from build123d import *

# Parameters (mm, degrees)
SKETCH1_R           = 2.5
BOSS_EXTRUDE1_DEPTH = 1
SKETCH2_R           = 1.5
BOSS_EXTRUDE2_DEPTH = 11.75
BOSS_EXTRUDE3_START = -12.75
SKETCH1_5_R         = 2.5
BOSS_EXTRUDE3_DEPTH = 1
FILLET1_R           = 0.05
SCALE1_SCALE        = 1.9


with BuildPart() as part:
    # Sketch1 → Boss-Extrude1 (new body)
    with BuildSketch(Plane.XY):
        Circle(SKETCH1_R)
    extrude(amount=-BOSS_EXTRUDE1_DEPTH)

    # Sketch2 → Boss-Extrude2 (add)
    with BuildSketch(Plane(origin=(0, 0, -1), x_dir=(-1, 0, 0), z_dir=(0, 0, -1))):
        Circle(SKETCH2_R)
    extrude(amount=BOSS_EXTRUDE2_DEPTH)

    # Sketch1<5> → Boss-Extrude3 (add)
    with BuildSketch(Plane.XY.offset(BOSS_EXTRUDE3_START)):
        Circle(SKETCH1_5_R)
    extrude(amount=-BOSS_EXTRUDE3_DEPTH)

    # Fillet1
    fillet1_edges = [part.edges().sort_by_distance(p)[0] for p in [
        (-2.5, 0, 0),
        (-2.5, 0, -1),
        (-2.5, 0, -12.75),
        (-2.5, 0, -13.75),
    ]]
    fillet(fillet1_edges, radius=FILLET1_R)


with BuildPart() as part_1:
    # Scale1: scaled about (0, 0, -6.875)
    add(part.part.scale(SCALE1_SCALE).moved(Location((0, 0, 6.1875))))


solid = part_1.part
Can you work these out from the model? Positions are in its coordinate system, mm. A direction names the side the tool comes from. Round coordinates to 2 decimals unless told otherwise and drop trailing zeros. Loops run counter-clockwise (first coordinate to the right, second up) from the corner with the lowest first, then second, coordinate; pieces in that order, holes last. Notation, with made-up numbers: (67, 54) - (107, 54) arc R24 cw to (107, 71) - close; hole circle Ø2 at (44, 77.5). An arc over 180 degrees is marked (long way). Write item = value, one per line. Start each with the question number.
(1) For faces 1 (the face through (0, 0, -19.938)), 2 (the face through (2.262, -1.734, -6.719)), which set-ups out of +Z, -Z, +X, -X, +Y, -Y let a thin tool reach every point of the face, with its end or its side?
(2) If I drill on probe 1 along Z at (x, y) = (3.5, -1); probe 2 along Y at (x, z) = (0, -16.25); probe 3 along X at (y, z) = (1.5, -6.75), over which ranges is the centre line in solid material (lowest first)? Write a range as [from, to].
(3) If we section it at C-C (z = -5.25): Please give me the cut outline in (x, y), and give its area (3 significant figures).
(4) For P1, Ø4, axis at y = -3, z = -11.5, coming from the -X side; P2, Ø1.5, axis at x = -2.5, z = -13.5, coming from the +Y side; P3, Ø3, axis at x = 1.5, z = 3, coming from the +Y side, each with a flat end and sliding along its axis, tell me the tip position at first contact or that it passes through.
Ans:
q1.face_1 = -Z, +X, -X, +Y, -Y
q1.face_2 = none
q2.probe_1 = [-19.94, -18.04], [4.29, 6.19]
q2.probe_2 = [-2.85, 2.85]
q2.probe_3 = [-2.42, 2.42]
q3.outline = circle Ø5.7 at (0, 0)
q3.area = 25.5 mm²
q4.P1 = -2.67
q4.P2 = 2.25
q4.P3 = 4.67
